```python
from build123d import *

# Parameters (mm, degrees)
SKETCH_1_W                  = 29.3
SKETCH_1_H                  = 13
EXTRUDE_1_DEPTH             = 7
SKETCH_2_W                  = 29.3
SKETCH_2_H                  = 8.4
EXTRUDE_2_DEPTH             = 4
SKETCH_3_W                  = 16.4
SKETCH_3_H                  = 7.4
SKETCH_3_W_2                = 15.4
SKETCH_3_H_2                = 6.4
SKETCH_3_W_3                = 7.4
SKETCH_3_R                  = 2.5
EXTRUDE_3_DEPTH             = 2
SKETCH_5_R                  = 1.4
EXTRUDE_4_DEPTH             = 5.8
CUT_EXTRUDE_1_DEPTH         = 5
SKETCH_7_R                  = 3.75
CUT_EXTRUDE_2_DEPTH         = 10
SKETCH_8_W                  = 10
SKETCH_8_H                  = 7
EXTRUDE_5_DEPTH             = 6.5
EXTRUDE_5_DIRECTION_2_REACH = 15


with BuildPart() as part:
    # 草图1 → 凸台-拉伸1 (new body)
    with BuildSketch(Plane(origin=(0, 0, 0), x_dir=(1, 0, 0), z_dir=(0, 1, 0))):
        Rectangle(SKETCH_1_W, SKETCH_1_H)
    extrude(amount=EXTRUDE_1_DEPTH)

    # 草图2 → 凸台-拉伸2 (add)
    with BuildSketch(Plane(origin=(0, 7, 0), x_dir=(1, 0, 0), z_dir=(0, 1, 0))):
        Rectangle(SKETCH_2_W, SKETCH_2_H)
    extrude(amount=EXTRUDE_2_DEPTH)

    # 草图3 → 凸台-拉伸3 (add)
    with BuildSketch(Plane(origin=(0, 11, 0), x_dir=(1, 0, 0), z_dir=(0, 1, 0))):
        with Locations((-5.95, 0)):
            Rectangle(SKETCH_3_W, SKETCH_3_H)
        with Locations((-5.95, 0)):
            Rectangle(SKETCH_3_W_2, SKETCH_3_H_2, mode=Mode.SUBTRACT)
        with Locations((10.45, 0)):
            Rectangle(SKETCH_3_W_3, SKETCH_3_H)
        with Locations((10.45, 0)):
            Circle(SKETCH_3_R, mode=Mode.SUBTRACT)
    extrude(amount=EXTRUDE_3_DEPTH)

    # 草图5 → 凸台-拉伸4 (add)
    with BuildSketch(Plane(origin=(0, 0, 0), x_dir=(1, 0, 0), z_dir=(0, 1, 0))):
        with BuildLine():
            Line((-18.5, 3.75), (18.5, 3.75))
            ThreePointArc((18.5, 3.75), (22.25, 0), (18.5, -3.75))
            Line((18.5, -3.75), (-18.5, -3.75))
            ThreePointArc((-18.5, -3.75), (-22.25, 0), (-18.5, 3.75))
        make_face()
        with Locations((18.5, 0)):
            Circle(SKETCH_5_R, mode=Mode.SUBTRACT)
        with Locations((-18.5, 0)):
            Circle(SKETCH_5_R, mode=Mode.SUBTRACT)
    extrude(amount=EXTRUDE_4_DEPTH)

    # 草图6 → 切除-拉伸1 (cut, symmetric)
    with BuildSketch(Plane.XY):
        Polygon((-22.25, 1.5), (-16.95, 1.5), (-16.95, 3.5), (-14.65, 5.8), (-22.25, 5.8), align=None)
        Polygon((22.25, 5.8), (22.25, 1.5), (16.95, 1.5), (16.95, 3.5), (14.65, 5.8), align=None)
    extrude(amount=CUT_EXTRUDE_1_DEPTH, both=True, mode=Mode.SUBTRACT)

    # 草图7 → 切除-拉伸2 (cut)
    with BuildSketch(Plane(origin=(0, 1.5, 0), x_dir=(1, 0, 0), z_dir=(0, 1, 0))):
        with Locations((18.5, 0)):
            Circle(SKETCH_7_R)
        with Locations((-18.5, 0)):
            Circle(SKETCH_7_R)
    extrude(amount=CUT_EXTRUDE_2_DEPTH, mode=Mode.SUBTRACT)

    # 草图8 → 凸台-拉伸5 (add)
    with BuildSketch(Plane(origin=(0, 0, -6.5), x_dir=(-1, 0, 0), z_dir=(0, 0, -1))):
        with Locations((0, 5.1)):
            Rectangle(SKETCH_8_W, SKETCH_8_H)
    extrude(amount=EXTRUDE_5_DEPTH)

    # 草图8 → 凸台-拉伸5 direction 2 (add, up to next)
    with BuildSketch(Plane(origin=(0, 0, -6.5), x_dir=(-1, 0, 0), z_dir=(0, 0, -1)), mode=Mode.PRIVATE) as extrude_5_direction_2_sk1:
        with Locations((0, 5.1)):
            Rectangle(SKETCH_8_W, SKETCH_8_H)
    extrude_5_direction_2_tool1 = extrude(extrude_5_direction_2_sk1.sketch, amount=-EXTRUDE_5_DIRECTION_2_REACH, mode=Mode.PRIVATE) - part.part
    add(extrude_5_direction_2_tool1.solids().sort_by_distance((0, 5.1, -6.5))[0])


solid = part.part
```
Source: CAD feature listing. Evaluate the final solid. Frame: model axes, mm. A direction names the side the tool comes from. Coordinates: 2 decimals unless noted, no trailing zeros. Loops run counter-clockwise (first coordinate to the right, second up) from the corner with the lowest first, then second, coordinate; pieces in that order, holes last. Notation, with made-up numbers: (-12.5, 7) -> (23.5, 7) arc R29 ccw to (23.5, 43) -> close; hole circle Ø7 at (26.25, 41). An arc over 180 degrees is marked (long way). One line per item, written item: value. Start each with the question number.
Q1. Section query D-D, the plane x = -19. Return the cut outline in (y, z), and give its area (3 significant figures).
Q2. Set-up query: faces 5 (the face through (-10, 7, -5)), 6 (the face through (10, 7, -5)), 7 (the face through (0, 1.6, -10)). Return all of +Z, -Z, +X, -X, +Y, -Y with unobstructed straight access to the full face (end or side cutting, diameter ignored); none if empty.
Q3. Mould query, pull axis X, two halves, no side actions, for faces 1 (the face through (1.75, 12, 0)), 2 (the face through (2.25, 12, 0)), 3 (the face through (22.25, 0.74, -0.08)), 4 (the face through (0, 7, 5)). Classes: pulls with the +X half, pulls with the -X half, needs draft (parallel to the pull), parting line crosses it, or undercut.
Q4. Line query: line 1 along X through (y, z) = (1, 0); line 2 along X through (y, z) = (12.75, 3); line 3 along X through (y, z) = (12.1, 0). Output: solid intervals per line, ascending.
Q5. Section query C-C, the plane z = -5.75. Return the cut outline in (x, y).
Q6. Section query A-A, the plane y = 2.75. Return the cut outline in (x, z).
Q7. Contact query for flat-ended pins moving along their axis: P1, Ø4, axis at x = 10.45, z = 0, coming from the -Y side; P2, Ø3.5, axis at x = -18.5, z = 0, coming from the +Y side; P3, Ø3, axis at x = -16, y = 2, coming from the -Z side; P4, Ø4, axis at x = 17, y = 3, coming from the +Z side. Output: stop coordinate, or through.
Q8. Section query B-B, the plane x = -2. Return the cut outline in (y, z), and give its area (3 significant figures).
Results:
1. outline: (0, -3.72) -> (1.5, -3.72) -> (1.5, -1.31) -> (0, -1.31) -> close; (0, 1.31) -> (1.5, 1.31) -> (1.5, 3.72) -> (0, 3.72) -> close
1. area: 7.23 mm^2
2. face 5: -Z, -X, +Y
2. face 6: -Z, +X, +Y
2. face 7: -Z, +X, -X, -Y
3. face 1: undercut
3. face 2: undercut
3. face 3: pulls with the +X half
3. face 4: needs draft
4. line 1: -22.25 to -19.9, -17.1 to 17.1, 19.9 to 22.25
4. line 2: -14.15 to -13.65, 1.75 to 2.25, 6.75 to 14.15
4. line 3: -14.15 to -13.65, 1.75 to 2.25, 6.75 to 7.95, 12.95 to 14.15
5. outline: (-14.65, 0) -> (14.65, 0) -> (14.65, 7) -> (5, 7) -> (5, 8.6) -> (-5, 8.6) -> (-5, 7) -> (-14.65, 7) -> close
6. outline: (-16.95, -3.75) -> (-14.65, -3.75) -> (-14.65, -6.5) -> (-5, -6.5) -> (-5, -13) -> (5, -13) -> (5, -6.5) -> (14.65, -6.5) -> (14.65, -3.75) -> (16.95, -3.75) -> (16.95, -3.41) arc R3.75 cw to (16.95, 3.41) -> (16.95, 3.75) -> (14.65, 3.75) -> (14.65, 6.5) -> (-14.65, 6.5) -> (-14.65, 3.75) -> (-16.95, 3.75) -> (-16.95, 3.41) arc R3.75 cw to (-16.95, -3.41) -> close
7. P1: y = 0
7. P2: y = 1.5
7. P3: z = -6.5
7. P4: z = 3.75
8. outline: (0, -6.5) -> (1.6, -6.5) -> (1.6, -13) -> (8.6, -13) -> (8.6, -4.2) -> (11, -4.2) -> (11, -3.7) -> (13, -3.7) -> (13, -3.2) -> (11, -3.2) -> (11, 3.2) -> (13, 3.2) -> (13, 3.7) -> (11, 3.7) -> (11, 4.2) -> (7, 4.2) -> (7, 6.5) -> (0, 6.5) -> close
8. area: 176 mm^2
